Geometry check sheet. Reference: the model listing, model coordinates, mm. Give positions to 0.01 mm unless a question says otherwise; leave off trailing zeros. Order: outer loops, then holes, each group sorted by start corner. A loop starts at its lowest first (then second) coordinate and runs counter-clockwise, first axis right, second up. Notation, with made-up numbers: M 36.5,41.25 L 57.5,41.25 A19 ccw 57.5,58.25 Z; hole C -13,71 d5. An arc over 180 degrees is marked long. Put each result on its own line as item: value. Start each with the question number.
Q1. Go/stop test with flat-tipped pins: pin 1 (2 mm diameter, centred on x = 45, z = -17.5, fed in from -Y); pin 2 (1 mm diameter, centred on x = 44.5, z = -4.5, fed in from -Y); pin 3 (3 mm diameter, centred on x = 28, z = -6, fed in from +Y). Record where each tip stops, or that it passes through.
Q2. Section check C-C on x = 20. Record the cut outline in (y, z).
Q3. Section check A-A on x = 89.5. Record the cut outline in (y, z).
Q4. Section check B-B on z = -24.5. Record the cut outline in (x, y).
Q5. Material ranges on L1, parallel to X at y = 46.5, z = -45; L2, parallel to Z at x = 30, y = 42; L3, parallel to Y at x = 67, z = -9, recorded low to high.
Q6. Mould release check, pull along X, two halves, no side actions. Record for faces 1 (the flat face through (0, 27, -24)), 2 (the flat face through (59, 2, 2)), 3 (the cylindrical face through (108.403, 46.085, -42.599)), 4 (the flat face through (25, 42, -39)): +X half, -X half, draft (parallel to the pull), parting line (faces both ways), or undercut.
```python
from build123d import *

# Parameters (mm, degrees)
SKETCH_1_W          = 120
SKETCH_1_H          = 73.539105243
SKETCH_1_R          = 1.8
SKETCH_1_W_2        = 48
SKETCH_1_H_2        = 31
SKETCH_1_W_3        = 23
SKETCH_1_H_3        = 2
SKETCH_1_W_4        = 7
SKETCH_1_H_4        = 7
SKETCH_1_H_5        = 7.044155877
EXTRUDE_1_DEPTH     = 5
SKETCH_2_W          = 37.5
SKETCH_2_H          = 36.110051057
CUT_EXTRUDE_1_DEPTH = 3.5


with BuildPart() as part:
    # Эскиз1 → Бобышка-Вытянуть1 (new body)
    with BuildSketch(Plane(origin=(0, 0, 0), x_dir=(1, 0, 0), z_dir=(0, 0.7071067811865477, 0.7071067811865475))):
        with Locations((60, 36.769552622)):
            Rectangle(SKETCH_1_W, SKETCH_1_H)
        with Locations(Location((10, 63.539105243, 0), (0, 0, 270))):
            Circle(SKETCH_1_R, mode=Mode.SUBTRACT)
        with Locations(Location((110, 63.539105243, 0), (0, 0, 270))):
            Circle(SKETCH_1_R, mode=Mode.SUBTRACT)
        with Locations(Location((110, 10, 0), (0, 0, 270))):
            Circle(SKETCH_1_R, mode=Mode.SUBTRACT)
        with Locations(Location((10, 10, 0), (0, 0, 270))):
            Circle(SKETCH_1_R, mode=Mode.SUBTRACT)
        with Locations((82, 36.5)):
            Rectangle(SKETCH_1_W_2, SKETCH_1_H_2, mode=Mode.SUBTRACT)
        with Locations((36.5, 57)):
            Rectangle(SKETCH_1_W_3, SKETCH_1_H_3, mode=Mode.SUBTRACT)
        with Locations((50.5, 47)):
            Rectangle(SKETCH_1_W_4, SKETCH_1_H_4, mode=Mode.SUBTRACT)
        with Locations((41, 47)):
            Rectangle(SKETCH_1_W_4, SKETCH_1_H_4, mode=Mode.SUBTRACT)
        with Locations((31.5, 47)):
            Rectangle(SKETCH_1_W_4, SKETCH_1_H_4, mode=Mode.SUBTRACT)
        with Locations((22, 47)):
            Rectangle(SKETCH_1_W_4, SKETCH_1_H_4, mode=Mode.SUBTRACT)
        with Locations((22, 38)):
            Rectangle(SKETCH_1_W_4, SKETCH_1_H_4, mode=Mode.SUBTRACT)
        Polygon((18.5, 32.5), (18.5, 25.455844123), (25.5, 25.5), (25.5, 32.5), align=None, mode=Mode.SUBTRACT)
        with Locations((22, 20)):
            Rectangle(SKETCH_1_W_4, SKETCH_1_H_4, mode=Mode.SUBTRACT)
        with Locations((31.5, 20)):
            Rectangle(SKETCH_1_W_4, SKETCH_1_H_4, mode=Mode.SUBTRACT)
        with Locations((41, 20)):
            Rectangle(SKETCH_1_W_4, SKETCH_1_H_4, mode=Mode.SUBTRACT)
        with Locations((50.5, 20)):
            Rectangle(SKETCH_1_W_4, SKETCH_1_H_4, mode=Mode.SUBTRACT)
        with Locations((50.5, 28.977922062)):
            Rectangle(SKETCH_1_W_4, SKETCH_1_H_5, mode=Mode.SUBTRACT)
        with Locations((41, 38)):
            Rectangle(SKETCH_1_W_4, SKETCH_1_H_4, mode=Mode.SUBTRACT)
        with Locations((50.5, 38)):
            Rectangle(SKETCH_1_W_4, SKETCH_1_H_4, mode=Mode.SUBTRACT)
        with Locations((31.5, 38)):
            Rectangle(SKETCH_1_W_4, SKETCH_1_H_4, mode=Mode.SUBTRACT)
        with Locations((31.5, 28.977922062)):
            Rectangle(SKETCH_1_W_4, SKETCH_1_H_5, mode=Mode.SUBTRACT)
        with Locations((41, 28.977922062)):
            Rectangle(SKETCH_1_W_4, SKETCH_1_H_5, mode=Mode.SUBTRACT)
    extrude(amount=EXTRUDE_1_DEPTH)

    # Фаска1
    # the kernel refuses this chamfer: 5.196152423, 3 mm, written as the material it takes off along each edge
    with BuildSketch(Plane(origin=(58, 18.384776311, -11.313708499), x_dir=(0.01932676561270104, -0.706974708221925, -0.7069747082219248), z_dir=(0, 0.7071067811865475, -0.7071067811865477)), Plane(origin=(106, 40.305086528, -33.234018716), x_dir=(-0.019326765612701025, -0.706974708221925, -0.7069747082219249), z_dir=(0, -0.7071067811865475, 0.7071067811865477))) as chamfer_1_piece_1:
        with BuildLine():
            Line((5.377156765, 0), (-0.239955173, 3.099864482))
            Line((-0.239955173, 3.099864482), (-0.343858811, 3.097855985))
            ThreePointArc((-0.343858811, 3.097855985), (-0.133898034, 1.549663153), (-0.103903638, -0.002008496))
            Line((-0.103903638, -0.002008496), (0.002008496, -0.103903638))
            ThreePointArc((0.002008496, -0.103903638), (2.689582631, -0.051951819), (5.379165261, -0.103903638))
            Line((5.379165261, -0.103903638), (5.377156765, 0))
        make_face()
    extrude(amount=31, mode=Mode.SUBTRACT)
    with BuildSketch(Plane(origin=(106, 18.384776311, -11.313708499), x_dir=(0, -0.6933086211987814, -0.7206407952450685), z_dir=(-1, 0, 0)), Plane(origin=(58, 40.305086528, -33.234018716), x_dir=(0, -0.7206407952450687, -0.693308621198781), z_dir=(1, 0, 0))) as chamfer_1_piece_2:
        with BuildLine():
            Line((5.377156765, 0), (-0.239955173, 3.099864482))
            Line((-0.239955173, 3.099864482), (-0.343858811, 3.097855985))
            ThreePointArc((-0.343858811, 3.097855985), (-0.133898034, 1.549663153), (-0.103903638, -0.002008496))
            Line((-0.103903638, -0.002008496), (0.002008496, -0.103903638))
            ThreePointArc((0.002008496, -0.103903638), (2.689582631, -0.051951819), (5.379165261, -0.103903638))
            Line((5.379165261, -0.103903638), (5.377156765, 0))
        make_face()
    extrude(amount=48, mode=Mode.SUBTRACT)
    with BuildSketch(Plane(origin=(106, 18.384776311, -11.313708499), x_dir=(0, -0.6933086211987814, -0.7206407952450685), z_dir=(-1, 0, 0))) as chamfer_1_piece_3a_section:
        with BuildLine():
            Line((5.377156765, 0), (-0.239955173, 3.099864482))
            Line((-0.239955173, 3.099864482), (-0.343858811, 3.097855985))
            ThreePointArc((-0.343858811, 3.097855985), (-0.133898034, 1.549663153), (-0.103903638, -0.002008496))
            Line((-0.103903638, -0.002008496), (0.002008496, -0.103903638))
            ThreePointArc((0.002008496, -0.103903638), (2.689582631, -0.051951819), (5.379165261, -0.103903638))
            Line((5.379165261, -0.103903638), (5.377156765, 0))
        make_face()
    chamfer_1_piece_3a = extrude(amount=61.442891912, mode=Mode.PRIVATE)
    chamfer_1_piece_3a = split(chamfer_1_piece_3a, bisect_by=Plane(origin=(58, 16.472259587, -11.865738078), z_dir=(-1, 0, 0)), keep=Keep.TOP, mode=Mode.PRIVATE)
    with BuildSketch(Plane(origin=(58, 8.879216281, -1.808148469), x_dir=(0.01932676561270103, -0.706974708221925, -0.7069747082219248), z_dir=(0, 0.7071067811865475, -0.7071067811865477))) as chamfer_1_piece_3b_section:
        with BuildLine():
            Line((5.377156765, 0), (-0.239955173, 3.099864482))
            Line((-0.239955173, 3.099864482), (-0.343858811, 3.097855985))
            ThreePointArc((-0.343858811, 3.097855985), (-0.133898034, 1.549663153), (-0.103903638, -0.002008496))
            Line((-0.103903638, -0.002008496), (0.002008496, -0.103903638))
            ThreePointArc((0.002008496, -0.103903638), (2.689582631, -0.051951819), (5.379165261, -0.103903638))
            Line((5.379165261, -0.103903638), (5.377156765, 0))
        make_face()
    chamfer_1_piece_3b = extrude(amount=44.442891912, mode=Mode.PRIVATE)
    chamfer_1_piece_3b = split(chamfer_1_piece_3b, bisect_by=Plane(origin=(57.037990314, 17.15250316, -12.54598165), z_dir=(0, -0.7071067811865475, 0.7071067811865477)), keep=Keep.TOP, mode=Mode.PRIVATE)
    chamfer_1_piece_3 = chamfer_1_piece_3a & chamfer_1_piece_3b
    add(chamfer_1_piece_3, mode=Mode.SUBTRACT)
    with BuildSketch(Plane(origin=(44.557108088, 40.305086528, -33.234018716), x_dir=(0, -0.7206407952450687, -0.693308621198781), z_dir=(1, 0, 0))) as chamfer_1_piece_4a_section:
        with BuildLine():
            Line((5.377156765, 0), (-0.239955173, 3.099864482))
            Line((-0.239955173, 3.099864482), (-0.343858811, 3.097855985))
            ThreePointArc((-0.343858811, 3.097855985), (-0.133898034, 1.549663153), (-0.103903638, -0.002008496))
            Line((-0.103903638, -0.002008496), (0.002008496, -0.103903638))
            ThreePointArc((0.002008496, -0.103903638), (2.689582631, -0.051951819), (5.379165261, -0.103903638))
            Line((5.379165261, -0.103903638), (5.377156765, 0))
        make_face()
    chamfer_1_piece_4a = extrude(amount=61.442891912, mode=Mode.PRIVATE)
    chamfer_1_piece_4a = split(chamfer_1_piece_4a, bisect_by=Plane(origin=(58, 39.753056949, -35.146535439), z_dir=(-1, 0, 0)), keep=Keep.TOP, mode=Mode.PRIVATE)
    with BuildSketch(Plane(origin=(58, 18.384776311, -11.313708499), x_dir=(0.01932676561270104, -0.706974708221925, -0.7069747082219248), z_dir=(0, 0.7071067811865475, -0.7071067811865477))) as chamfer_1_piece_4b_section:
        with BuildLine():
            Line((5.377156765, 0), (-0.239955173, 3.099864482))
            Line((-0.239955173, 3.099864482), (-0.343858811, 3.097855985))
            ThreePointArc((-0.343858811, 3.097855985), (-0.133898034, 1.549663153), (-0.103903638, -0.002008496))
            Line((-0.103903638, -0.002008496), (0.002008496, -0.103903638))
            ThreePointArc((0.002008496, -0.103903638), (2.689582631, -0.051951819), (5.379165261, -0.103903638))
            Line((5.379165261, -0.103903638), (5.377156765, 0))
        make_face()
    chamfer_1_piece_4b = extrude(amount=44.442891912, mode=Mode.PRIVATE)
    chamfer_1_piece_4b = split(chamfer_1_piece_4b, bisect_by=Plane(origin=(57.037990314, 39.072813376, -34.466291867), z_dir=(0, 0.7071067811865475, -0.7071067811865477)), keep=Keep.TOP, mode=Mode.PRIVATE)
    chamfer_1_piece_4 = chamfer_1_piece_4a & chamfer_1_piece_4b
    add(chamfer_1_piece_4, mode=Mode.SUBTRACT)
    with BuildSketch(Plane(origin=(106, 40.305086528, -33.234018716), x_dir=(-0.019326765612701025, -0.706974708221925, -0.7069747082219249), z_dir=(0, -0.7071067811865475, 0.7071067811865477))) as chamfer_1_piece_5a_section:
        with BuildLine():
            Line((5.377156765, 0), (-0.239955173, 3.099864482))
            Line((-0.239955173, 3.099864482), (-0.343858811, 3.097855985))
            ThreePointArc((-0.343858811, 3.097855985), (-0.133898034, 1.549663153), (-0.103903638, -0.002008496))
            Line((-0.103903638, -0.002008496), (0.002008496, -0.103903638))
            ThreePointArc((0.002008496, -0.103903638), (2.689582631, -0.051951819), (5.379165261, -0.103903638))
            Line((5.379165261, -0.103903638), (5.377156765, 0))
        make_face()
    chamfer_1_piece_5a = extrude(amount=44.442891912, mode=Mode.PRIVATE)
    chamfer_1_piece_5a = split(chamfer_1_piece_5a, bisect_by=Plane(origin=(106.962009686, 17.15250316, -12.54598165), z_dir=(0, -0.7071067811865475, 0.7071067811865477)), keep=Keep.TOP, mode=Mode.PRIVATE)
    with BuildSketch(Plane(origin=(119.442891912, 18.384776311, -11.313708499), x_dir=(0, -0.6933086211987812, -0.7206407952450685), z_dir=(-1, 0, 0))) as chamfer_1_piece_5b_section:
        with BuildLine():
            Line((5.377156765, 0), (-0.239955173, 3.099864482))
            Line((-0.239955173, 3.099864482), (-0.343858811, 3.097855985))
            ThreePointArc((-0.343858811, 3.097855985), (-0.133898034, 1.549663153), (-0.103903638, -0.002008496))
            Line((-0.103903638, -0.002008496), (0.002008496, -0.103903638))
            ThreePointArc((0.002008496, -0.103903638), (2.689582631, -0.051951819), (5.379165261, -0.103903638))
            Line((5.379165261, -0.103903638), (5.377156765, 0))
        make_face()
    chamfer_1_piece_5b = extrude(amount=61.442891912, mode=Mode.PRIVATE)
    chamfer_1_piece_5b = split(chamfer_1_piece_5b, bisect_by=Plane(origin=(106, 16.472259587, -11.865738078), z_dir=(1, 0, 0)), keep=Keep.TOP, mode=Mode.PRIVATE)
    chamfer_1_piece_5 = chamfer_1_piece_5a & chamfer_1_piece_5b
    add(chamfer_1_piece_5, mode=Mode.SUBTRACT)
    with BuildSketch(Plane(origin=(58, 40.305086528, -33.234018716), x_dir=(0, -0.7206407952450687, -0.693308621198781), z_dir=(1, 0, 0))) as chamfer_1_piece_6a_section:
        with BuildLine():
            Line((5.377156765, 0), (-0.239955173, 3.099864482))
            Line((-0.239955173, 3.099864482), (-0.343858811, 3.097855985))
            ThreePointArc((-0.343858811, 3.097855985), (-0.133898034, 1.549663153), (-0.103903638, -0.002008496))
            Line((-0.103903638, -0.002008496), (0.002008496, -0.103903638))
            ThreePointArc((0.002008496, -0.103903638), (2.689582631, -0.051951819), (5.379165261, -0.103903638))
            Line((5.379165261, -0.103903638), (5.377156765, 0))
        make_face()
    chamfer_1_piece_6a = extrude(amount=61.442891912, mode=Mode.PRIVATE)
    chamfer_1_piece_6a = split(chamfer_1_piece_6a, bisect_by=Plane(origin=(106, 39.753056949, -35.146535439), z_dir=(1, 0, 0)), keep=Keep.TOP, mode=Mode.PRIVATE)
    with BuildSketch(Plane(origin=(106, 49.810646557, -42.739578745), x_dir=(-0.019326765612701025, -0.706974708221925, -0.7069747082219249), z_dir=(0, -0.7071067811865475, 0.7071067811865477))) as chamfer_1_piece_6b_section:
        with BuildLine():
            Line((5.377156765, 0), (-0.239955173, 3.099864482))
            Line((-0.239955173, 3.099864482), (-0.343858811, 3.097855985))
            ThreePointArc((-0.343858811, 3.097855985), (-0.133898034, 1.549663153), (-0.103903638, -0.002008496))
            Line((-0.103903638, -0.002008496), (0.002008496, -0.103903638))
            ThreePointArc((0.002008496, -0.103903638), (2.689582631, -0.051951819), (5.379165261, -0.103903638))
            Line((5.379165261, -0.103903638), (5.377156765, 0))
        make_face()
    chamfer_1_piece_6b = extrude(amount=44.442891912, mode=Mode.PRIVATE)
    chamfer_1_piece_6b = split(chamfer_1_piece_6b, bisect_by=Plane(origin=(106.962009686, 39.072813376, -34.466291867), z_dir=(0, 0.7071067811865475, -0.7071067811865477)), keep=Keep.TOP, mode=Mode.PRIVATE)
    chamfer_1_piece_6 = chamfer_1_piece_6a & chamfer_1_piece_6b
    add(chamfer_1_piece_6, mode=Mode.SUBTRACT)

    # Эскиз2 → Вырез-Вытянуть1 (cut)
    with BuildSketch(Plane(origin=(0, 0, 0), x_dir=(1, 0, 0), z_dir=(0, 0.7071067811865477, 0.7071067811865475))):
        with Locations((36.25, 33.597850417)):
            Rectangle(SKETCH_2_W, SKETCH_2_H)
    extrude(amount=CUT_EXTRUDE_1_DEPTH, mode=Mode.SUBTRACT)


solid = part.part
```
Results found:
1. pin 1: stops at y = 21.45
1. pin 2: stops at y = 4
1. pin 3: stops at y = 14.57
2. outline: M 0,0 L 10.99,-10.99 L 13.47,-8.52 L 14.14,-9.19 L 15.2,-8.13 L 3.54,3.54 Z; M 19.09,-14.14 L 20.48,-15.53 L 21.54,-14.47 L 20.15,-13.08 Z; M 25.46,-20.51 L 26.87,-21.92 L 27.93,-20.86 L 26.52,-19.45 Z; M 31.82,-26.87 L 33.23,-28.28 L 34.29,-27.22 L 32.88,-25.81 Z; M 36.52,-36.52 L 52,-52 L 55.54,-48.46 L 39.24,-32.17 L 38.18,-33.23 L 39,-34.05 Z
3. outline: M 0,0 L 14.77,-14.77 L 16.26,-9.19 L 3.54,3.54 Z; M 36.85,-36.85 L 52,-52 L 55.54,-48.46 L 42.43,-35.36 Z
4. outline: M 0,24.5 L 17.5,24.5 L 17.5,29.45 L 18.5,29.45 L 18.5,31.57 L 0,31.57 Z; M 25.5,29.45 L 28,29.45 L 28,31.57 L 25.5,31.57 Z; M 35,29.45 L 37.5,29.45 L 37.5,31.57 L 35,31.57 Z; M 44.5,29.45 L 47,29.45 L 47,31.57 L 44.5,31.57 Z; M 54,29.45 L 55,29.45 L 55,24.5 L 57.89,24.5 L 55,31.57 L 54,31.57 Z; M 106.11,24.5 L 120,24.5 L 120,31.57 L 109,31.57 Z
5. L1: x = 0 to 8.62, 11.38 to 108.62, 111.38 to 120
5. L2: z = -42 to -40.02, -37.2 to -34.93
5. L3: y = 9 to 16.07
6. face 1: -X half
6. face 2: draft
6. face 3: undercut
6. face 4: undercut
